Could you check a few things on this drawing? It's one solid part, dimensions in mm from its lowest x, y, z. A direction names the side the tool comes from. Give positions to 0.01 mm unless a question says otherwise; leave off trailing zeros. Loops run counter-clockwise (first coordinate to the right, second up) from the corner with the lowest first, then second, coordinate; pieces in that order, holes last.
1. Imagine slicing it at D-D (y = 6.15). List the corners of the cut face in (x, z) for me, plus the area to 3 significant figures.
2. Imagine slicing it at C-C (x = 14.1). List the corners of the cut face in (y, z) for me, plus the area to 3 significant figures.
3. Imagine slicing it at B-B (x = 11.6). List the corners of the cut face in (y, z) for me.
4. For P1, Ø3, axis at x = 5, y = 3.5, coming from the -Z side, with a flat end and sliding along its axis, tell me the tip position at first contact or that it passes through.
5. I need wall thicknesses on line 1 along Z through (x, y) = (3.5, 12); line 2 along X through (y, z) = (6, 1); line 3 along X through (y, z) = (6.75, 2.25). Which ranges of each line are inside material? Lowest first, please.
6. Thinking about a two-plate mould opening in Y: for the marked faces 3, 4, 5 and 6, which applies, +Y half, -Y half, draft (parallel to the pull), parting line (faces both ways), or undercut?
7. For the marked faces 1 and 2, which set-ups out of +Z, -Z, +X, -X, +Y, -Y let a thin tool reach every point of the face, with its end or its side?
8. Imagine slicing it at A-A (y = 11.15). List the corners of the cut face in (x, z) for me.
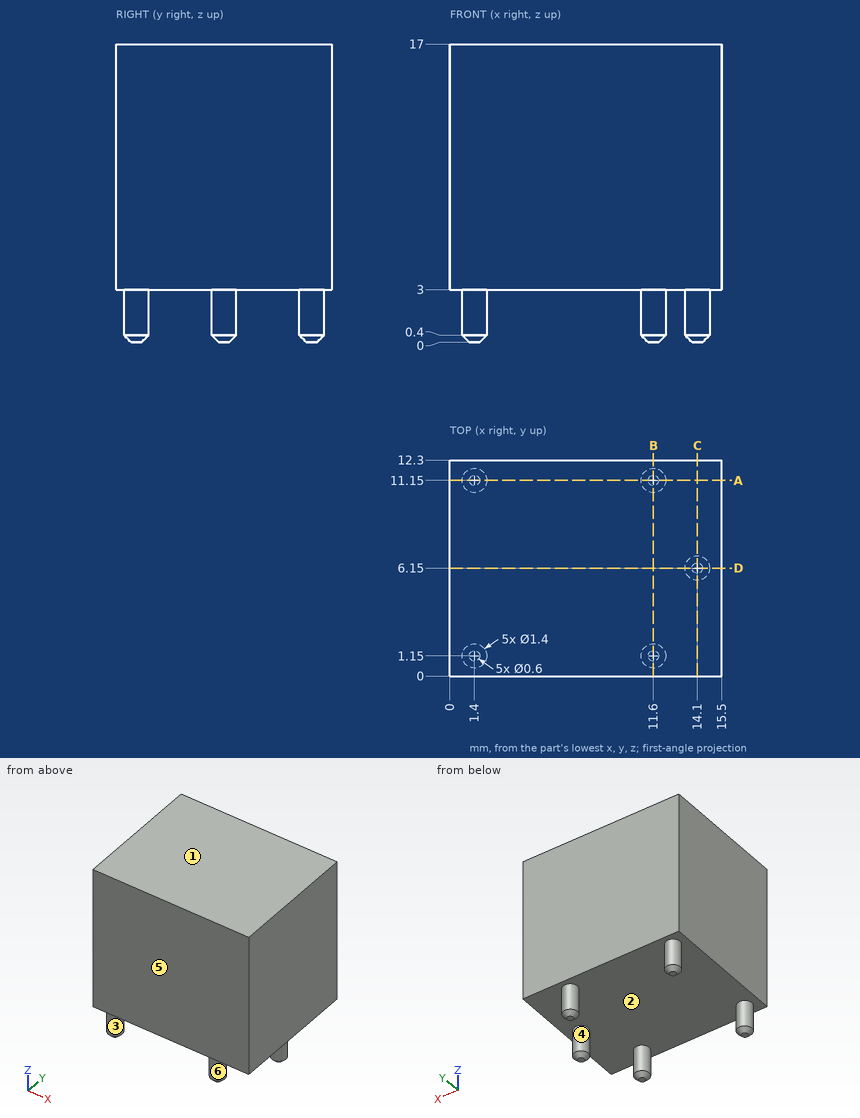
Derived:
1. outline: (0, 3) - (13.4, 3) - (13.4, 0.4) - (13.8, 0) - (14.4, 0) - (14.8, 0.4) - (14.8, 3) - (15.5, 3) - (15.5, 17) - (0, 17) - close
1. area: 221 mm2
2. outline: (0, 3) - (5.45, 3) - (5.45, 0.4) - (5.85, 0) - (6.45, 0) - (6.85, 0.4) - (6.85, 3) - (12.3, 3) - (12.3, 17) - (0, 17) - close
2. area: 176 mm2
3. outline: (0, 3) - (0.45, 3) - (0.45, 0.4) - (0.85, 0) - (1.45, 0) - (1.85, 0.4) - (1.85, 3) - (10.45, 3) - (10.45, 0.4) - (10.85, 0) - (11.45, 0) - (11.85, 0.4) - (11.85, 3) - (12.3, 3) - (12.3, 17) - (0, 17) - close
4. P1: stops at z = 3
5. line 1: z = 3 to 17
5. line 2: x = 13.42 to 14.78
5. line 3: x = 13.74 to 14.46
6. face 3: undercut
6. face 4: parting line
6. face 5: -Y half
6. face 6: undercut
7. face 1: +Z, +X, -X, +Y, -Y
7. face 2: -Z
8. outline: (0, 3) - (0.7, 3) - (0.7, 0.4) - (1.1, 0) - (1.7, 0) - (2.1, 0.4) - (2.1, 3) - (10.9, 3) - (10.9, 0.4) - (11.3, 0) - (11.9, 0) - (12.3, 0.4) - (12.3, 3) - (15.5, 3) - (15.5, 17) - (0, 17) - close
